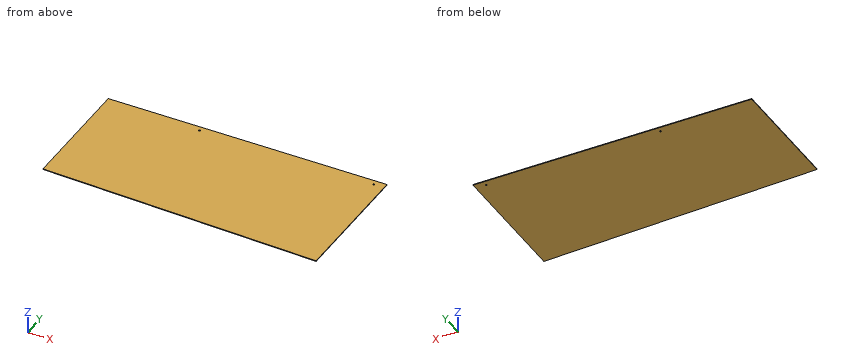
```python
from build123d import *

# Parameters (mm, degrees)
SKETCH1_W           = 80
SKETCH1_H           = 35
SKETCH1_R           = 0.25
BOSS_EXTRUDE4_DEPTH = 0.2
BOSS_EXTRUDE5_DEPTH = 0.2


with BuildPart() as part:
    # Sketch1 → Boss-Extrude4 (new body)
    with BuildSketch(Plane.XY):
        with Locations((8.187411056, -3.455555556)):
            Rectangle(SKETCH1_W, SKETCH1_H)
        with Locations((-4.812588944, 12.544444444)):
            Circle(SKETCH1_R, mode=Mode.SUBTRACT)
        with Locations((45.187411056, 12.544444444)):
            Circle(SKETCH1_R, mode=Mode.SUBTRACT)
    extrude(amount=BOSS_EXTRUDE4_DEPTH)

    # Sketch3 → Boss-Extrude5 (add)
    with BuildSketch(Plane.XY.offset(0.2)):
        Polygon((-31.812588944, -20.955555556), (48.187411056, -23.955555556), (48.187411056, -20.955555556), align=None)
    extrude(amount=-BOSS_EXTRUDE5_DEPTH)


solid = part.part
```
CAD build for the part. Positions are in the model's coordinates, mm. Give positions to 0.01 mm unless a question says otherwise; leave off trailing zeros. Order: outer loops, then holes, each group sorted by start corner. A loop starts at its lowest first (then second) coordinate and runs counter-clockwise, first axis right, second up.
(1) Saw through at B-B, the plane x = 26.5. Give the cut face in (y, z).
(2) Saw through at C-C, the plane x = 9. Give the cut face in (y, z), then the cut area to 3 significant figures.
(3) Saw through at A-A, the plane z = 0.1. Give the cut face in (x, y), then the cut area to 3 significant figures.
(4) Drill centre lines: L1, parallel to Y at x = 37.5, z = 0.15; L2, parallel to Y at x = -22, z = 0.1. Where is each one in solid material? Low to high.
Results found:
1. outline: (-23.14, 0) - (14.04, 0) - (14.04, 0.2) - (-23.14, 0.2) - close
2. outline: (-22.49, 0) - (14.04, 0) - (14.04, 0.2) - (-22.49, 0.2) - close
2. area: 7.31 mm2
3. outline: (-31.81, -20.96) - (48.19, -23.96) - (48.19, 14.04) - (-31.81, 14.04) - close; hole circle Ø0.5 at (-4.81, 12.54); hole circle Ø0.5 at (45.19, 12.54)
3. area: 2,920 mm2
4. L1: y = -23.55 to 14.04
4. L2: y = -21.32 to 14.04
